Model file for the job. Use its own axes, mm. A direction names the side the tool comes from. Round coordinates to 2 decimals unless told otherwise and drop trailing zeros. Loops run counter-clockwise (first coordinate to the right, second up) from the corner with the lowest first, then second, coordinate; pieces in that order, holes last. Notation, with made-up numbers: (82.5, 61.5) -> (99.5, 61.5) arc R25 cw to (99.5, 77.5) -> close; hole circle Ø8 at (-39, 69). An arc over 180 degrees is marked (long way). Use a Markdown table: item, result. Add a question column.
Autodesk Inventor part; units mm, degrees
ref_plane "Work Plane1" through (0, 0, -20) normal (0, 0, -1) x (0, 1, 0)
ref_plane "Work Plane3" through (0, 0.51, -6) normal (0, 0, -1) x (0, 1, 0)
ref_plane "YZ Plane" through (0, 0, 0) normal (1, 0, 0) x (0, 1, 0)
sketch "Sketch1" plane through (0, 0, 0) normal (0, 0, 1) x (1, 0, 0)
  line L0 (36, 0.51) -> (25.6472, -38.1271)
  line L1 (36, 0.51) -> (76, 0.51) construction
  line L2 (36, 0.51) -> (25.6472, -38.1271) construction
  line L3 (25.6472, -38.1271) -> (30.4769, -39.4212)
  line L4 (30.4769, -39.4212) -> (40.8296, -0.7841)
  line L5 (40.8296, -0.7841) -> (36, 0.51)
  line L6 (36, 0.51) -> (40.8296, -0.7841)
  line L7 (40.8296, -0.7841) -> (44.7119, 13.7048)
  line L8 (44.7119, 13.7048) -> (39.8823, 14.9989)
  line L9 (39.8823, 14.9989) -> (36, 0.51)
  arc A0 (36, -1.5) -> (26, 8.5) centre (26, -1.5) ccw construction
  line L10 (39.0787, 12) -> (34.0787, 12)
  line L11 (34.0787, 12) -> (34.0787, 9)
  line L12 (34.0787, 9) -> (38.2749, 9)
  line L13 (14, -12.5) -> (26, -12.5) construction
  line L14 (0, -20) -> (30.5044, -20)
  line L15 (30.5044, -20) -> (35.8634, 0)
  line L16 (35.1935, -2.5) -> (0, -2.5)
  line L17 (35.1935, -2.5) -> (30.5044, -20)
  line L18 (0, -20) -> (0, -2.5)
  line L19 (-41.5, -2.5) -> (36, -2.5) construction
  line L20 (30.5044, -20) -> (35.1935, -2.5) construction
  point P0 (0, 0)
  point P1 (17.5967, -2.5)
  dimension "d0" = 40
  dimension "d1" = 105
  dimension "d2" = 5
  dimension "d3" = 15
  dimension "d5" = 5
  dimension "d6" = 3
  dimension "d7" = 11.49
  dimension "d20" = 17.5
  dimension "d21" = 35.1935
  dimension "d22" = 30.5044
ref_plane "Work Plane1" through (0, 0, -20) normal (0, 0, -1) x (0, 1, 0)
extrude "Extrusion1" add sketch "Sketch1" against normal up to surface (20 mm away) contours L5 L4 L3 L0 | L9 L8 L7 L5 | L0 L14 L18 L16
ref_plane "Work Plane6" through (36, 0, -14) normal (0, 0, 1) x (1, 0, 0)
ref_plane "Work Plane3" through (0, 0.51, -6) normal (0, 0, -1) x (0, 1, 0)
fillet "Fillet2" radius 10 1 edges at (30.5044, -20, -10)
chamfer "Chamfer1" distance 12 angle 45 1 edges at (0, -20, -10)
properties part number "Stand_Back"
1) Cut at C-C on y = -25. Write the cut outline in (x, z), and give its area (3 significant figures).
2) Tool access for faces 5 (the face through (18, -2.5, -10)), 6 (the face through (15, -20, -10)), 7 (the face through (24, -10, 0)): list every direction of +Z, -Z, +X, -X, +Y, -Y with a clear straight run to the whole face (end or side of a thin tool).
3) Wall check: probe 1 along Y at (x, z) = (16, -4.75); probe 2 along X at (y, z) = (-30.5, -7); probe 3 along Y at (x, z) = (8, -12). Give the ranges that are in metal, low to high. Write a range as from..to.
4) Pull direction Y, two halves, no side cores. Call faces 1 (the face through (26.4, -35.32, -9.86)), 2 (the face through (25.327, -23.811, -10.14)), 3 (the face through (42.331, 14.343, -9.86)), 4 (the face through (28.028, -38.765, -9.86)): +Y half, -Y half, draft (parallel to the pull), parting line (faces both ways), or undercut.
5) Cut at B-B on x = 15. Write the cut outline in (y, z).
6) Cut at A-A on z = -15.5. Write the cut outline in (x, y), and give its area (3 significant figures).
7) Pin check, flat tips, straight feed: pin 1 Ø3 at (y, z) = (-23.5, -17) entering from -X; pin 2 Ø4 at (y, z) = (2.5, -17.5) entering from -X; pin 3 Ø12 at (y, z) = (-33, -8) entering from -X. Stop position of each tip, or through.
Established:
| question | item | result |
|---|---|---|
| 1 | outline | (26.13, -20) -> (34.34, -20) -> (34.34, 0) -> (26.13, 0) -> close |
| 1 | area | 164 mm^2 |
| 2 | face 5 | +Z, -Z, -X, +Y |
| 2 | face 6 | +Z, -Z, -X, -Y |
| 2 | face 7 | +Z, +X, -X, +Y, -Y |
| 3 | probe 1 | y = -20..-2.5 |
| 3 | probe 2 | x = 27.46..32.87 |
| 3 | probe 3 | y = -16..-2.5 |
| 4 | face 1 | undercut |
| 4 | face 2 | undercut |
| 4 | face 3 | +Y half |
| 4 | face 4 | -Y half |
| 5 | outline | (-20, -20) -> (-2.5, -20) -> (-2.5, 0) -> (-20, 0) -> close |
| 6 | outline | (0, -8) -> (12, -20) -> (17.47, -20) arc R10 cw to (27.13, -32.59) -> (25.65, -38.13) -> (30.48, -39.42) -> (40.83, -0.78) -> (44.71, 13.7) -> (39.88, 15) -> (36, 0.51) -> (35.19, -2.5) -> (0, -2.5) -> close |
| 6 | area | 817 mm^2 |
| 7 | pin 1 | stops at x = 23.47 |
| 7 | pin 2 | stops at x = 36 |
| 7 | pin 3 | stops at x = 25.65 |
